from build123d import *

# Parameters (mm, degrees)
SCALE1_SCALE = 25.4


with BuildPart() as part:
    # Sketch1 → Revolve-Thin2 (revolve)
    with BuildSketch(Plane(origin=(0, 0, 0), x_dir=(0, 0, -1), z_dir=(1, 0, 0))):
        with BuildLine():
            ThreePointArc((19.195710728, 0), (18.051167415, 9.914732181), (14.677744268, 19.307916406))
            ThreePointArc((14.677744268, 19.307916406), (11.557742765, 22.742167977), (7.095710728, 24.014474279))
            Line((7.095710728, 24.014474279), (7.095710728, 23.914474279))
            ThreePointArc((7.095710728, 23.914474279), (11.505002693, 22.657206311), (14.588126579, 19.263546712))
            ThreePointArc((14.588126579, 19.263546712), (17.953797581, 9.891948074), (19.095710728, 0))
            Line((19.095710728, 0), (19.095610728, 0))
            ThreePointArc((19.095610728, 0), (17.953700211, 9.891925289), (14.588036962, 19.263502342))
            ThreePointArc((14.588036962, 19.263502342), (11.504907472, 22.657147719), (7.095610728, 23.914374278))
            Line((7.095610728, 23.914374278), (7.095610728, 24.014574278))
            ThreePointArc((7.095610728, 24.014574278), (11.557753024, 22.742279309), (14.677833886, 19.307960776))
            ThreePointArc((14.677833886, 19.307960776), (18.051264784, 9.914754965), (19.195810728, 0))
            Line((19.195810728, 0), (19.195710728, 0))
        make_face()
    revolve(axis=Axis((0, 0, -7.095710728), (0, 0, 1)))


with BuildPart() as part_1:
    # Scale1: scaled about (0, 1e-09, -13.921880613)
    add(part.part.scale(SCALE1_SCALE).moved(Location((0, -2.4e-08, 339.693886957))))


solid = part_1.part
The model under review builds one solid part; all positions refer to its coordinate system, in mm. Coordinates: 2 decimals unless noted, no trailing zeros. Write each loop counter-clockwise with the first axis right and the second up, starting at its lowest first coordinate (ties: lowest second). Pieces come first, ordered by that corner, then holes. Notation, with made-up numbers: (-33.75, 44.25) - (-19.75, 44.25) arc R31 ccw to (-19.75, 72.25) - close; hole circle Ø9 at (70.5, 61.5). An arc over 180 degrees is marked (long way). Answer as a JSON object with one key per item and string values. Group by question number.
1. Add section A-A (z = 71). Give the boundary of the cut face in (x, y).
2. Clearance check with flat-ended pins moving along their axes: pin 1 Ø4 at (x, y) = (243.5, -287) entering from +Z; pin 2 Ø1.5 at (x, y) = (161.5, 107.5) entering from +Z; pin 3 Ø6 at (x, y) = (-5, 239.5) entering from +Z. State where each tip first meets the part, or that it passes through.
3. Add section B-B (z = -67.5). Give the boundary of the cut face in (x, y).
Findings:
{
 "1": {"outline": "circle Ø1181.84 at (0, 0); circle Ø1176.25 at (0, 0); hole circle Ø1181.83 at (0, 0); hole circle Ø1176.24 at (0, 0)"},
 "2": {"pin 1": "z = -78.39", "pin 2": "z = -128", "pin 3": "z = -118.33"},
 "3": {"outline": "circle Ø827.59 at (0, 0); circle Ø813.91 at (0, 0); hole circle Ø827.58 at (0, 0); hole circle Ø813.9 at (0, 0)"}
}
